Source: CAD feature listing. Evaluate the final solid. Frame: model axes, mm. A direction names the side the tool comes from. Give positions to 0.01 mm unless a question says otherwise; leave off trailing zeros. Write each loop counter-clockwise with the first axis right and the second up, starting at its lowest first coordinate (ties: lowest second). Pieces come first, ordered by that corner, then holes. Notation, with made-up numbers: (25, 75) -> (54, 75) arc R29 cw to (54, 114) -> close; hole circle Ø8 at (-2.5, 56.5). An arc over 180 degrees is marked (long way). Use one line per item in the form item = value. Start each with the question number.
(1) Cut plane B-B, the plane x = 145.5. Output: boundary loops of the cut face in (y, z).
(2) Set-up query: faces 4 (the face through (106.52, 3.76, 98.8)), 5 (the face through (8.242, 3.757, 54.723)), 6 (the face through (-10.207, 4, 167)), 7 (the face through (97.57, 3.86, 24.62)). Return all of +Z, -Z, +X, -X, +Y, -Y with unobstructed straight access to the full face (end or side cutting, diameter ignored); none if empty.
(3) Cut plane A-A, the plane z = 53. Output: boundary loops of the cut face in (x, y).
(4) Cut plane D-D, the plane y = 2.25. Count the separate pieces of the cut face and the enclosed holes in it, and give its area (3 significant figures).
(5) Material intervals for line 1 along X through (y, z) = (3.25, 88); line 2 along Z through (x, y) = (11.5, 3); line 3 along Z through (x, y) = (80, 4), sorted ascending. Write a range as from..to.
(6) Cut plane C-C, the plane x = 95. Output: boundary loops of the cut face in (y, z), and give its area (3 significant figures).
(7) Draft query along X for faces 1 (the face through (-49.29, 3.76, 129.16)), 2 (the face through (105.738, 3.757, 111.317)), 3 (the face through (-3.432, 3.757, 172.974)). Return one class per face: pulls with the +X half, pulls with the -X half, needs draft (parallel to the pull), parting line crosses it, or undercut.
(8) First-contact query: P1, Ø2, axis at y = 5, z = 167, coming from the -X side; P2, Ø1.5, axis at y = 3.5, z = 81.5, coming from the +X side; P3, Ø2, axis at y = 5, z = 168.5, coming from the +X side. Flat tips, straight axial feed; report the tip coordinate or a pass-through.
from build123d import *

# Parameters (mm, degrees)
SKETCH3_R           = 2.5
SKETCH3_R_2         = 52.3875
SKETCH3_R_3         = 3.3
SKETCH3_R_4         = 4.5
SKETCH3_R_5         = 27.4955
SKETCH3_R_6         = 3.300000004
BOSS_EXTRUDE1_DEPTH = 7.62
CUT_EXTRUDE3_REACH  = 321.448
CUT_EXTRUDE4_REACH  = 321.448
FILLET1_R           = 6.35
CUT_EXTRUDE10_REACH = 321.448
CUT_EXTRUDE12_REACH = 321.448
CUT_EXTRUDE15_START = -7.62
CUT_EXTRUDE15_DEPTH = 7.62


# Read off the part's stored shape, not the designer's step: Cut-Extrude15
with BuildPart() as part:
    # Sketch3 → Boss-Extrude1 (new body)
    with BuildSketch(Plane(origin=(0, 0, 0), x_dir=(-1, 0, 0), z_dir=(0, 1, 0))):
        with BuildLine():
            Line((-49.427109136, 17.679572239), (34.112309331, 92.818281558))
            ThreePointArc((34.112309331, 92.818281558), (49.260131818, 129.740728466), (29.825562347, 164.597881552))
            ThreePointArc((29.825562347, 164.597881552), (28.145398332, 165.051242365), (26.567761736, 164.316701751))
            Line((26.567761736, 164.316701751), (21.302878118, 159.051818133))
            ThreePointArc((21.302878118, 159.051818133), (14.21924173, 157.642795249), (10.20668404, 163.648012211))
            Line((10.20668404, 163.648012211), (10.20668404, 170.220745001))
            ThreePointArc((10.20668404, 170.220745001), (9.549518747, 171.925600851), (7.91807501, 172.748273949))
            ThreePointArc((7.91807501, 172.748273949), (3.367898451, 172.974), (-1.182278109, 172.748273949))
            ThreePointArc((-1.182278109, 172.748273949), (-2.813721846, 171.925600851), (-3.470887139, 170.220745001))
            Line((-3.470887139, 170.220745001), (-3.470887139, 163.648012211))
            ThreePointArc((-3.470887139, 163.648012211), (-9.970887139, 157.148012211), (-16.470887139, 163.648012211))
            Line((-16.470887139, 163.648012211), (-16.470887139, 164.225022653))
            ThreePointArc((-16.470887139, 164.225022653), (-17.760387302, 166.435870942), (-20.319588051, 166.401924563))
            Line((-20.319588051, 166.401924563), (-168.403592651, 158.863977372))
            Line((-168.403592651, 158.863977372), (-265.178957518, 163.648012211))
            Line((-265.178957518, 163.648012211), (-268.446360693, 19.778758396))
            ThreePointArc((-268.446360693, 19.778758396), (-265.639755471, 12.584633122), (-258.423714062, 9.834866275))
            Line((-258.423714062, 9.834866275), (-55.796807523, 15.236419982))
            ThreePointArc((-55.796807523, 15.236419982), (-52.385720802, 15.868157792), (-49.427109136, 17.679572239))
        make_face()
        with Locations(Location((-168.403592651, 39.801477371, 0), (0, 0, 90))):
            Circle(SKETCH3_R, mode=Mode.SUBTRACT)
        with Locations(Location((-225.553592651, 96.951477371, 0), (0, 0, 90))):
            Circle(SKETCH3_R, mode=Mode.SUBTRACT)
        with Locations(Location((-168.403592651, 96.951477372, 0), (0, 0, 90))):
            Circle(SKETCH3_R_2, mode=Mode.SUBTRACT)
        with Locations(Location((-111.253592651, 96.951477371, 0), (0, 0, 90))):
            Circle(SKETCH3_R, mode=Mode.SUBTRACT)
        with Locations(Location((-168.403592651, 154.101477371, 0), (0, 0, 90))):
            Circle(SKETCH3_R, mode=Mode.SUBTRACT)
        with Locations(Location((-55.796807523, 24.761419982, 0), (0, 0, 90))):
            Circle(SKETCH3_R_3, mode=Mode.SUBTRACT)
        with Locations(Location((28.436615228, 156.875733282, 0), (0, 0, 90))):
            Circle(SKETCH3_R_4, mode=Mode.SUBTRACT)
        with Locations(Location((-9.970887139, 90.351987789, 0), (0, 0, 90))):
            Circle(SKETCH3_R_4, mode=Mode.SUBTRACT)
        with Locations(Location((16.70668404, 90.351987789, 0), (0, 0, 90))):
            Circle(SKETCH3_R_4, mode=Mode.SUBTRACT)
        with Locations(Location((-30.407092297, 107.5, 0), (0, 0, 90))):
            Circle(SKETCH3_R_4, mode=Mode.SUBTRACT)
        with Locations(Location((37.142889198, 107.5, 0), (0, 0, 90))):
            Circle(SKETCH3_R_4, mode=Mode.SUBTRACT)
        with Locations(Location((3.367898451, 127, 0), (0, 0, 90))):
            Circle(SKETCH3_R_5, mode=Mode.SUBTRACT)
        with Locations(Location((-35.039603917, 133.772278929, 0), (0, 0, 90))):
            Circle(SKETCH3_R_4, mode=Mode.SUBTRACT)
        with Locations(Location((41.775400818, 133.772278929, 0), (0, 0, 90))):
            Circle(SKETCH3_R_4, mode=Mode.SUBTRACT)
        with Locations(Location((-21.700818327, 156.875733282, 0), (0, 0, 90))):
            Circle(SKETCH3_R_4, mode=Mode.SUBTRACT)
        with Locations(Location((3.367898451, 166, 0), (0, 0, 90))):
            Circle(SKETCH3_R_4, mode=Mode.SUBTRACT)
        with Locations(Location((-258.931181349, 19.346338398, 0), (0, 0, 90))):
            Circle(SKETCH3_R_6, mode=Mode.SUBTRACT)
    extrude(amount=BOSS_EXTRUDE1_DEPTH)

    # Sketch12 → Cut-Extrude3 (cut, up to next)
    with BuildSketch(Plane(origin=(0, 7.62, 0), x_dir=(1, 0, 0), z_dir=(0, 1, 0)), mode=Mode.PRIVATE) as cut_extrude3_sk1:
        with BuildLine():
            Line((265.178957518, -163.648012211), (267.97556459, -40.508702148))
            Line((267.97556459, -40.508702148), (230.316092651, -96.951477372))
            ThreePointArc((230.316092651, -96.951477372), (212.182341242, -140.730225962), (168.403592651, -158.863977372))
            Line((168.403592651, -158.863977372), (265.178957518, -163.648012211))
        make_face()
    cut_extrude3_tool1 = extrude(cut_extrude3_sk1.sketch, amount=-CUT_EXTRUDE3_REACH, mode=Mode.PRIVATE) & part.part
    # Sketch12 → Cut-Extrude3 (cut, up to next)
    with BuildSketch(Plane(origin=(0, 7.62, 0), x_dir=(1, 0, 0), z_dir=(0, 1, 0)), mode=Mode.PRIVATE) as cut_extrude3_sk2:
        with BuildLine():
            Line((267.97556459, -40.508702148), (268.273601144, -27.385651725))
            Line((268.273601144, -27.385651725), (228.792351717, -83.300271022))
            ThreePointArc((228.792351717, -83.300271022), (229.933978242, -90.083486013), (230.316092651, -96.951477372))
            Line((230.316092651, -96.951477372), (267.97556459, -40.508702148))
        make_face()
    cut_extrude3_tool2 = extrude(cut_extrude3_sk2.sketch, amount=-CUT_EXTRUDE3_REACH, mode=Mode.PRIVATE) & part.part
    add(cut_extrude3_tool1.solids().sort_by_distance((242.898488, 7.62, 120.934583))[0], mode=Mode.SUBTRACT)
    add(cut_extrude3_tool2.solids().sort_by_distance((248.238841, 7.62, 62.857625))[0], mode=Mode.SUBTRACT)

    # Sketch13 → Cut-Extrude4 (cut, up to next)
    with BuildSketch(Plane(origin=(0, 7.62, 0), x_dir=(1, 0, 0), z_dir=(0, 1, 0)), mode=Mode.PRIVATE) as cut_extrude4_sk1:
        Polygon((205.359295361, -30.862514021), (251.718937312, -10.013599753), (60.814888047, -15.102649833), (135.412495886, -34.423028757), align=None)
    cut_extrude4_tool1 = extrude(cut_extrude4_sk1.sketch, amount=-CUT_EXTRUDE4_REACH, mode=Mode.PRIVATE) & part.part
    add(cut_extrude4_tool1.solids().sort_by_distance((160.937928, 7.62, 21.113641))[0], mode=Mode.SUBTRACT)

    # Fillet1
    fillet1_edges = [part.edges().sort_by_distance(p)[0] for p in [
        (268.273601144, 3.81, 27.385651725),
        (228.792351717, 3.81, 83.300271022),
        (205.359295361, 3.81, 30.862514021),
        (135.412495886, 3.81, 34.423028757),
        (60.814888047, 3.81, 15.102649833),
        (251.718937312, 3.81, 10.013599753),
        (258.423714062, 3.81, 9.834866275),
        (268.446360693, 3.81, 19.778758396),
    ]]
    fillet(fillet1_edges, radius=FILLET1_R)

    # Sketch14 → Cut-Extrude10 (cut, up to next)
    with BuildSketch(Plane(origin=(0, 7.62, 0), x_dir=(1, 0, 0), z_dir=(0, 1, 0)), mode=Mode.PRIVATE) as cut_extrude10_sk1:
        with BuildLine():
            Line((244.52170499, -20.212940115), (207.524518121, -36.851359757))
            ThreePointArc((207.524518121, -36.851359757), (203.733724344, -42.021157152), (206.219824449, -47.930152738))
            ThreePointArc((206.219824449, -47.930152738), (214.983198468, -56.165475138), (221.98921849, -65.939570631))
            ThreePointArc((221.98921849, -65.939570631), (227.324020713, -69.178317741), (232.928793139, -66.433117629))
            Line((232.928793139, -66.433117629), (256.310542684, -33.319129513))
            ThreePointArc((256.310542684, -33.319129513), (257.474332837, -28.977686692), (255.544041259, -24.91856022))
            Line((255.544041259, -24.91856022), (251.895986311, -21.657423526))
            ThreePointArc((251.895986311, -21.657423526), (248.438629388, -19.762105057), (244.52170499, -20.212940115))
        make_face()
    cut_extrude10_tool1 = extrude(cut_extrude10_sk1.sketch, amount=-CUT_EXTRUDE10_REACH, mode=Mode.PRIVATE) & part.part
    add(cut_extrude10_tool1.solids().sort_by_distance((231.191654, 7.62, 42.620708))[0], mode=Mode.SUBTRACT)

    # Sketch19 → Cut-Extrude12 (cut, up to next)
    with BuildSketch(Plane(origin=(0, 7.62, 0), x_dir=(1, 0, 0), z_dir=(0, 1, 0)), mode=Mode.PRIVATE) as cut_extrude12_sk1:
        with BuildLine():
            Line((69.235394101, -23.843032422), (125.774906007, -38.486461693))
            ThreePointArc((125.774906007, -38.486461693), (130.483030138, -43.330085475), (128.351144664, -49.739624343))
            ThreePointArc((128.351144664, -49.739624343), (118.321232933, -60.552096865), (111.133194535, -73.43001577))
            ThreePointArc((111.133194535, -73.43001577), (108.875130187, -76.266983385), (105.448899127, -77.453651229))
            Line((105.448899127, -77.453651229), (8.811557915, -82.372799497))
            ThreePointArc((8.811557915, -82.372799497), (7.906607304, -82.355788757), (7.012785778, -82.213282427))
            ThreePointArc((7.012785778, -82.213282427), (5.382114006, -81.866354479), (3.739935744, -81.578778428))
            ThreePointArc((3.739935744, -81.578778428), (-1.488167541, -77.00545388), (0.396861915, -70.320020062))
            Line((0.396861915, -70.320020062), (43.530504975, -31.52388852))
            ThreePointArc((43.530504975, -31.52388852), (47.329210716, -29.879304731), (51.350676973, -30.860441973))
            Line((51.350676973, -30.860441973), (52.480075426, -31.573618446))
            ThreePointArc((52.480075426, -31.573618446), (56.613803862, -31.757331678), (60.021401634, -29.410048407))
            Line((60.021401634, -29.410048407), (62.404331593, -26.234763269))
            ThreePointArc((62.404331593, -26.234763269), (65.456340654, -24.000636026), (69.235394101, -23.843032422))
        make_face()
    cut_extrude12_tool1 = extrude(cut_extrude12_sk1.sketch, amount=-CUT_EXTRUDE12_REACH, mode=Mode.PRIVATE) & part.part
    add(cut_extrude12_tool1.solids().sort_by_distance((66.631089, 7.62, 56.211545))[0], mode=Mode.SUBTRACT)

    # Cut-Extrude15 outline → Cut-Extrude15 (cut)
    with BuildSketch(Plane(origin=(0, 7.62, 0), x_dir=(1, 0, 0), z_dir=(0, 1, 0)).offset(CUT_EXTRUDE15_START)):
        with BuildLine():
            ThreePointArc((40.660849974, -140.231703904), (39.001844492, -144.844146352), (36.861191377, -149.253741431))
            ThreePointArc((36.861191377, -149.253741431), (37.035613438, -155.845233628), (42.881616461, -158.895223973))
            Line((42.881616461, -158.895223973), (123.520323562, -154.790457105))
            ThreePointArc((123.520323562, -154.790457105), (129.329486204, -150.437715141), (127.48704531, -143.416451383))
            ThreePointArc((127.48704531, -143.416451383), (119.32579193, -134.694385747), (112.991346909, -124.567427074))
            ThreePointArc((112.991346909, -124.567427074), (110.452063443, -121.853539717), (106.841075413, -120.973817853))
            Line((106.841075413, -120.973817853), (62.446585261, -123.233638711))
            ThreePointArc((62.446585261, -123.233638711), (60.509103742, -123.633603237), (58.781566428, -124.597668114))
            Line((58.781566428, -124.597668114), (42.892536771, -136.97318668))
            ThreePointArc((42.892536771, -136.97318668), (41.523311936, -138.428909918), (40.660849974, -140.231703904))
        make_face()
        with BuildLine():
            ThreePointArc((32.229200226, -97.90609614), (32.230013577, -97.907091323), (32.2308269, -97.908086529))
            ThreePointArc((32.2308269, -97.908086529), (32.963651262, -98.668536238), (33.809910067, -99.300328325))
            Line((33.809910067, -99.300328325), (58.274621766, -114.638670821))
            ThreePointArc((58.274621766, -114.638670821), (60.09112394, -115.422332807), (62.059204559, -115.623491788))
            Line((62.059204559, -115.623491788), (101.082626056, -113.637075421))
            ThreePointArc((101.082626056, -113.637075421), (105.786794259, -111.258015784), (107.181907879, -106.174436215))
            ThreePointArc((107.181907879, -106.174436215), (106.515656468, -98.695326918), (106.759699387, -91.190567769))
            ThreePointArc((106.759699387, -91.190567769), (104.979666567, -86.085957931), (99.954945116, -84.091532504))
            Line((99.954945116, -84.091532504), (36.935219874, -87.299437113))
            ThreePointArc((36.935219874, -87.299437113), (31.322143272, -91.156322431), (32.229200226, -97.90609614))
        make_face()
    extrude(amount=CUT_EXTRUDE15_DEPTH, mode=Mode.SUBTRACT)


solid = part.part
Geometry says:
q1.outline = (0, 33.91) -> (7.62, 33.91) -> (7.62, 49.84) -> (0, 49.84) -> close; (0, 144.07) -> (7.62, 144.07) -> (7.62, 160.03) -> (0, 160.03) -> close
q2.face_4 = +Y, -Y
q2.face_5 = -Z, -X, +Y, -Y
q2.face_6 = +Z, +Y, -Y
q2.face_7 = -Z, +Y, -Y
q3.outline = (10.16, 0) -> (19.65, 0) -> (19.65, 7.62) -> (10.16, 7.62) -> close; (124.8, 0) -> (139.9, 0) -> (139.9, 7.62) -> (124.8, 7.62) -> close; (196.91, 0) -> (212.01, 0) -> (212.01, 7.62) -> (196.91, 7.62) -> close; (242.41, 0) -> (250.19, 0) -> (250.19, 7.62) -> (242.41, 7.62) -> close
q4.separate_pieces = 1
q4.enclosed_holes = 21
q4.area = 11,800 mm^2
q5.line_1 = -28.76..-20.54, -12.87..6.13, 13.81..34.31, 106.25..116.79, 220.02..229.67
q5.line_2 = 51.79..60.33, 82.24..86.12, 94.58..103.87, 150.13..157.33
q5.line_3 = 20.07..26.63, 78.75..85.11, 114.71..122.34, 157.01..163.36
q6.outline = (0, 23.96) -> (7.62, 23.96) -> (7.62, 30.52) -> (0, 30.52) -> close; (0, 77.99) -> (7.62, 77.99) -> (7.62, 84.34) -> (0, 84.34) -> close; (0, 113.95) -> (7.62, 113.95) -> (7.62, 121.58) -> (0, 121.58) -> close; (0, 156.24) -> (7.62, 156.24) -> (7.62, 162.6) -> (0, 162.6) -> close
q6.area = 205 mm^2
q7.face_1 = pulls with the -X half
q7.face_2 = undercut
q7.face_3 = parting line crosses it
q8.P1 = -10.21
q8.P2 = 230.59
q8.P3 = 3.47
